Geometry: final body of the model. Coordinates: model frame, mm. A direction names the side the tool comes from. Give positions to 0.01 mm unless a question says otherwise; leave off trailing zeros. Write each loop counter-clockwise with the first axis right and the second up, starting at its lowest first coordinate (ties: lowest second). Pieces come first, ordered by that corner, then holes. Notation, with made-up numbers: (2, 77.5) -> (50, 77.5) arc R22 cw to (50, 105.5) -> close; hole circle Ø1 at (2.5, 15). An arc over 180 degrees is marked (long way). Use CSV: the item, a comma, the result in double quotes. Start each with the question number.
1) Section B-B (x = 26). Output: boundary loops of the cut face in (y, z).
2) Draft query along X for faces 1 (the face through (37.195, -0.267, 0.633)), 2 (the face through (0, 0, 0)), 3 (the face through (0, 0, 1.588)). Return one class per face: pulls with the +X half, pulls with the -X half, needs draft (parallel to the pull), parting line crosses it, or undercut.
3) Set-up query: faces 4 (the face through (-37.467, -0.267, -3.921)), 5 (the face through (-51, 0, -3.238)), 6 (the face through (-51, 0, -4.826)), 7 (the face through (51, 0, -3.238)). Return all of +Z, -Z, +X, -X, +Y, -Y with unobstructed straight access to the full face (end or side cutting, diameter ignored); none if empty.
4) Material intervals for line 1 (Z direction, x = 29, y = 12.5); line 2 (Z direction, x = 54, y = -7.5); line 3 (X direction, y = -13.5, z = -3.5), sorted ascending. Write a range as [from, to].
5) Contact query for flat-ended pins moving along their axis: P1, Ø11, axis at x = -56.5, y = -6.5, coming from the +Z side; P2, Ø11.5, axis at x = 14.5, y = -8, coming from the -Z side; P3, Ø1, axis at y = -3, z = -2.5, coming from the +X side. Output: stop coordinate, or through.
Autodesk Inventor part; units mm, degrees
ref_plane "YZ Plane" through (0, 0, 0) normal (1, 0, 0) x (0, 1, 0)
ref_plane "XZ Plane" through (0, 0, 0) normal (0, 1, 0) x (-1, 0, 0)
ref_plane "XY Plane" through (0, 0, 0) normal (0, 0, 1) x (1, 0, 0)
sketch "Sketch1" plane through (0, 0, 0) normal (0, 0, 1) x (1, 0, 0)
  line L0 (-38.1, -19.05) -> (38.1, -19.05)
  line L1 (38.1, -19.05) -> (38.1, 19.05)
  line L2 (38.1, 19.05) -> (-38.1, 19.05)
  line L3 (-38.1, 19.05) -> (-38.1, -19.05)
  line L4 (-38.1, -19.05) -> (38.1, 19.05) construction
  line L5 (38.1, -19.05) -> (-38.1, 19.05) construction
  point P0 (0, 0)
  dimension "d0" = 76.2
  dimension "d1" = 38.1
extrude "Plate1" add sketch "Sketch1" along normal blind 1.5875
sketch "Sketch2" plane through (36.5125, -19.05, 1.5875) normal (1, 0, 0) x (0, 1, 0)
  line L0 (38.1, 0) -> (0, 0)
  line L1 (0, 0) -> (0, -4.826)
  line L2 (0, -4.826) -> (38.1, -4.826)
  line L3 (38.1, -4.826) -> (38.1, 0)
edge flange "Flange1" height 4.826 angle 90 thickness 1.5875 bend radius 1.5875 thickness toward (1, 0, 0) relief tear relief width 1.5875 relief depth 0.7937 corner gap 1.5875 corner form 0 edges at (38.1, 0, 0) (-38.1, 0, 0) wall of the first edge with corners at (36.5125, 19.05, 1.5875) (36.5125, -19.05, 1.5875) (36.5125, -19.05, -3.2385) (36.5125, 19.05, -3.2385)
bend "Bend1"
corner "Corner1"
sketch "Sketch3" plane through (-38.1, -19.05, -3.2385) normal (0, 0, -1) x (-1, 0, 0)
  line L0 (0, 38.1) -> (0, 0)
  line L1 (0, 0) -> (23.8125, 0)
  line L2 (23.8125, 0) -> (23.8125, 38.1)
  line L3 (23.8125, 38.1) -> (0, 38.1)
edge flange "Flange2" height 25.4 angle 90 thickness 1.5875 bend radius 1.5875 thickness toward (0, 0, -1) relief tear relief width 1.5875 relief depth 0.7937 corner gap 1.5875 corner form 0 edges at (-38.1, 0, -3.2385) (38.1, 0, -3.2385) wall of the first edge with corners at (-38.1, 19.05, -3.2385) (-38.1, -19.05, -3.2385) (-61.9125, -19.05, -3.2385) (-61.9125, 19.05, -3.2385)
bend "Bend2"
corner "Corner2"
fillet "Fillet1" radius 6.35 4 edges at (-61.9125, 19.05, -4.0323) (-61.9125, -19.05, -4.0323) (61.9125, -19.05, -4.0323) (61.9125, 19.05, -4.0323)
equation "\"d3\" = BendReliefWidth"
equation "\"d4\" = BendReliefDepth"
equation "\"d5\" = MinimumRemnant"
equation "\"d6\" = BendRadius"
equation "\"d9\" = BendRadius"
equation "\"d10\" = CornerReliefSize"
equation "\"d11\" = GapSize"
equation "\"d12\" = JacobiRadiusSize"
equation "\"d13\" = BendReliefWidth"
equation "\"d14\" = BendReliefDepth"
equation "\"d15\" = MinimumRemnant"
equation "\"d16\" = BendRadius"
equation "\"d19\" = BendRadius"
equation "\"d20\" = CornerReliefSize"
equation "\"d21\" = GapSize"
equation "\"d22\" = JacobiRadiusSize"
equation "\"BendRadius\" = Thickness"
equation "\"BendReliefWidth\" = Thickness"
equation "\"BendReliefDepth\" = 0.5 * Thickness"
equation "\"CornerReliefSize\" = 4 * Thickness"
equation "\"MinimumRemnant\" = 2 * Thickness"
equation "\"TransitionRadius\" = BendRadius"
equation "\"JacobiRadiusSize\" = BendRadius"
equation "\"GapSize\" = Thickness"
equation "\"d2\" = BendRadius"
properties part number "Center Rail Bracket" material "Steel, Galvanized"
Answers follow:
1,outline,"(-19.05, 0) -> (19.05, 0) -> (19.05, 1.59) -> (-19.05, 1.59) -> close"
2,face 1,"pulls with the +X half"
2,face 2,"undercut"
2,face 3,"needs draft"
3,face 4,"-Z, +Y, -Y"
3,face 5,"+Z, -X, +Y, -Y"
3,face 6,"-Z, +X, -X, +Y, -Y"
3,face 7,"+Z, +X, +Y, -Y"
4,line 1,"z = [0, 1.59]"
4,line 2,"z = [-4.83, -3.24]"
4,line 3,"x = [-61.86, -37.11], [37.11, 61.86]"
5,P1,"stops at z = -3.24"
5,P2,"stops at z = 0"
5,P3,"stops at x = 38.85"
